Check sheet for the modelled part. Datum: model origin and axes. Units: mm. A direction names the side the tool comes from. Give positions to 0.01 mm unless a question says otherwise; leave off trailing zeros. Loops run counter-clockwise (first coordinate to the right, second up) from the corner with the lowest first, then second, coordinate; pieces in that order, holes last. Notation, with made-up numbers: (-12, 48.25) - (42, 48.25) arc R26 ccw to (42, 87.25) - close; hole circle Ø4 at (26.5, 70.25). An arc over 180 degrees is marked (long way). Answer in a Markdown table with one row per item. Add a question column.
(1) Go/stop test with flat-tipped pins: P1, Ø5, axis at x = 38, y = 4.5, coming from the +Z side; P2, Ø5, axis at y = 9.5, z = -2, coming from the +X side. Record where each tip stops, or that it passes through.
(2) Sectioned sample at B-B on y = 9.75. Enter the section's corners in (x, z).
(3) Draft check along X on faces 4 (the face through (35, 12, 0)), 5 (the face through (0, 5, -5)), 6 (the face through (40, 5, -5)). Enter one of: released by +X, released by -X, zero draft, split by the parting line, or undercut.
(4) Thickness scan on L1, parallel to Y at x = 31.5, z = -7.5; L2, parallel to Y at x = 37.5, z = -7; L3, parallel to X at y = 7.5, z = -7.75. Record the ranges inside material, lowest first.
(5) Sectioned sample at A-A on x = 31.5. Enter the section's corners in (y, z).
(6) Set-up check for faces 1 (the face through (58.455, 13.455, -4.93)), 2 (the face through (17, 12.5, -5)), 3 (the face through (35, 8, -5)): record each of +Z, -Z, +X, -X, +Y, -Y from which the full face is reachable in a straight line by a thin tool's end or side.
(7) Sectioned sample at C-C on x = 3.5. Enter the section's corners in (y, z).
(8) Sectioned sample at D-D on z = -6. State how many separate pieces and enclosed holes the cut face has, then the cut area to 3 significant figures.
from build123d import *

# Parameters (mm, degrees)
CROQUIS1_R              = 1
SALIENTE_EXTRUIR1_DEPTH = 10
SALIENTE_EXTRUIR2_DEPTH = 10
REDONDEO1_R             = 1
REDONDEO2_R             = 6


with BuildPart() as part:
    # Croquis1 → Saliente-Extruir1 (new body)
    with BuildSketch(Plane.XY):
        Polygon((0, 0), (6, 0), (6, 12.5), (29, 12.5), (29, 0), (35, 0), (35, 16.5), (0, 16.5), align=None)
        with Locations((3.5, 6.25)):
            Circle(CROQUIS1_R, mode=Mode.SUBTRACT)
        with Locations((31.5, 6.25)):
            Circle(CROQUIS1_R, mode=Mode.SUBTRACT)
    extrude(amount=-SALIENTE_EXTRUIR1_DEPTH)

    # Croquis4 → Saliente-Extruir2 (add, through all)
    with BuildSketch(Plane.XY):
        with BuildLine():
            Line((45, 11.5), (35, 11.5))
            Line((35, 11.5), (35, 16.5))
            Line((35, 16.5), (45, 16.5))
            ThreePointArc((45, 16.5), (58.975424859, 13.200849719), (70, 4))
            ThreePointArc((70, 4), (65.603760626, 0.546008902), (60.016254104, 0.354316441))
            ThreePointArc((60.016254104, 0.354316441), (52.480888042, 1.331572321), (45, 0))
            Line((45, 0), (35, 0))
            Line((35, 0), (35, 5))
            Line((35, 5), (44.209457127, 5))
            ThreePointArc((44.209457127, 5), (52.795894624, 6.337270923), (61.405382505, 5.157473974))
            ThreePointArc((61.405382505, 5.157473974), (61.84041484, 5.057582168), (62.283868073, 5.006781226))
            ThreePointArc((62.283868073, 5.006781226), (54.231657294, 9.823135811), (45, 11.5))
        make_face()
    extrude(amount=-SALIENTE_EXTRUIR2_DEPTH)

    # Redondeo1
    redondeo1_edges = [part.edges().sort_by_distance(p)[0] for p in [
        (70, 4, -5),
    ]]
    fillet(redondeo1_edges, radius=REDONDEO1_R)

    # Redondeo2
    redondeo2_edges = [part.edges().sort_by_distance(p)[0] for p in [
        (0, 16.5, -5),
    ]]
    fillet(redondeo2_edges, radius=REDONDEO2_R)


solid = part.part
Reply:
| question | item | result |
|---|---|---|
| 1 | P1 | z = 0 |
| 1 | P2 | x = 67.44 |
| 2 | outline | (0, -10) - (6, -10) - (6, 0) - (0, 0) - close; (29, -10) - (35, -10) - (35, 0) - (29, 0) - close; (54.42, -10) - (64.4, -10) - (64.4, 0) - (54.42, 0) - close |
| 3 | face 4 | zero draft |
| 3 | face 5 | released by -X |
| 3 | face 6 | undercut |
| 4 | L1 | 0 to 5.25, 7.25 to 16.5 |
| 4 | L2 | 0 to 5, 11.5 to 16.5 |
| 4 | L3 | 0 to 6, 29 to 35, 58.93 to 66.94 |
| 5 | outline | (0, -10) - (5.25, -10) - (5.25, 0) - (0, 0) - close; (7.25, -10) - (16.5, -10) - (16.5, 0) - (7.25, 0) - close |
| 6 | face 1 | +Z, -Z, +X, +Y |
| 6 | face 2 | +Z, -Z, -Y |
| 6 | face 3 | +Z, -Z |
| 7 | outline | (0, -10) - (5.25, -10) - (5.25, 0) - (0, 0) - close; (7.25, -10) - (15.95, -10) - (15.95, 0) - (7.25, 0) - close |
| 8 | separate pieces | 1 |
| 8 | enclosed holes | 3 |
| 8 | area | 610 mm^2 |
